Verification items for this drawing (mm, ordinates from the low corner). Coordinates: 2 decimals unless noted, no trailing zeros. Order: outer loops, then holes, each group sorted by start corner. A loop starts at its lowest first (then second) coordinate and runs counter-clockwise, first axis right, second up. Notation, with made-up numbers: M -34.5,50 L 20.5,50 A22 ccw 20.5,59 Z; hole C 33.25,13.25 d9. An arc over 180 degrees is marked long. Answer as a JSON object with one key per item and string values. Group by question number.
(1) Cross-section at D-D (z = 47). Enter the section's corners in (x, y).
(2) Cross-section at B-B (z = 3.75). Enter the section's corners in (x, y).
(3) Cross-section at C-C (x = 3.75). Enter the section's corners in (y, z).
(4) Cross-section at A-A (y = 3.25). Enter the section's corners in (x, z), plus the area to 3 significant figures.
(5) Material ranges on line 1 (X direction, y = 2.8, z = 3.75); line 2 (Z direction, x = 3.75, y = 5); line 3 (Y direction, x = 16, z = 82.5), recorded low to high.
(6) Mould release check, pull along X, two halves, no side actions. Record for the marked faces 1 and 2: released by +X, released by -X, zero draft, split by the parting line, or undercut.
(7) Gauge pin test, flat ends, axial feed: pin 1 Ø4 at (x, z) = (28.5, 24) entering from +Y; pin 2 Ø3 at (x, z) = (3.75, 86.25) entering from -Y. Record the tip position at first contact, or that the pin passes through.
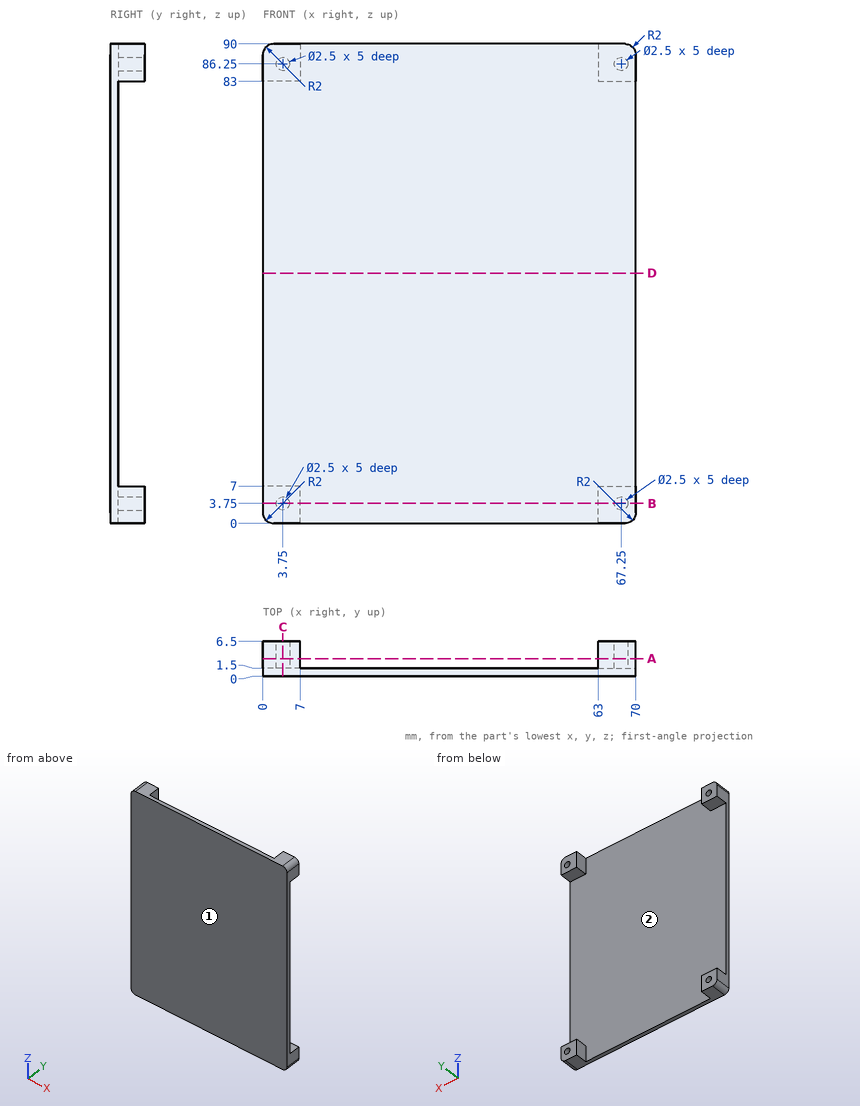
Taken from the geometry:
{
 "1": {"outline": "M 0,0 L 70,0 L 70,1.5 L 0,1.5 Z"},
 "2": {"outline": "M 0,0 L 70,0 L 70,6.5 L 68.5,6.5 L 68.5,1.5 L 66,1.5 L 66,6.5 L 63,6.5 L 63,1.5 L 7,1.5 L 7,6.5 L 5,6.5 L 5,1.5 L 2.5,1.5 L 2.5,6.5 L 0,6.5 Z"},
 "3": {"outline": "M 0,0 L 6.5,0 L 6.5,2.5 L 1.5,2.5 L 1.5,5 L 6.5,5 L 6.5,7 L 1.5,7 L 1.5,83 L 6.5,83 L 6.5,85 L 1.5,85 L 1.5,87.5 L 6.5,87.5 L 6.5,90 L 0,90 Z"},
 "4": {"outline": "M 0,2 A2 ccw 2,0 L 7,0 L 7,7 L 0,7 Z; M 0,83 L 7,83 L 7,90 L 2,90 A2 ccw 0,88 Z; M 63,0 L 68,0 A2 ccw 70,2 L 70,7 L 63,7 Z; M 63,83 L 70,83 L 70,88 A2 ccw 68,90 L 63,90 Z; hole C 3.75,3.75 d2.5; hole C 3.75,86.25 d2.5; hole C 67.25,3.75 d2.5; hole C 67.25,86.25 d2.5", "area": "173 mm²"},
 "5": {"line 1": "x = 0 to 2.5, 5 to 7, 63 to 66, 68.5 to 70", "line 2": "z = 0 to 2.5, 5 to 7, 83 to 85, 87.5 to 90", "line 3": "y = 0 to 1.5"},
 "6": {"face 1": "zero draft", "face 2": "undercut"},
 "7": {"pin 1": "stops at y = 1.5", "pin 2": "stops at y = 0"}
}
